CAD build for the part. Positions are in the model's coordinates, mm. Face numbers are marked on the shaded views. A direction names the side the tool comes from. Round coordinates to 2 decimals unless told otherwise and drop trailing zeros. Loops run counter-clockwise (first coordinate to the right, second up) from the corner with the lowest first, then second, coordinate; pieces in that order, holes last. Notation, with made-up numbers: (13, -16) - (31, -16) arc R4 cw to (31, -12) - close; hole circle Ø1 at (2.25, -20). An arc over 180 degrees is marked (long way). Use one line per item in the form item = value.
from build123d import *

# Parameters (mm, degrees)
F1_DEPTH       = 15
F3_DEPTH       = 112.001
F5_DEPTH       = 5
F7_DEPTH       = 112
F9_DEPTH       = 25
F12_DEPTH      = 15
F12_DEPTH_BACK = 5
F14_DEPTH      = 25
F15_R          = 3


# Not quite as in the source:
# - a pattern or mirror of a feature is missing from the dataset's text; its kind, count and spacing are read off the source's solid


with BuildPart() as f1:
    # F0 (on Top) → F1 (new body)
    with BuildSketch(Plane.XY):
        with BuildLine():
            Line((-56, 50), (-56, 0))
            Line((-56, 0), (56, 0))
            Line((56, 0), (56, 50))
            Line((56, 50), (36, 50))
            ThreePointArc((36, 50), (0, 14), (-36, 50))
            Line((-36, 50), (-56, 50))
        make_face()
    extrude(amount=F1_DEPTH)

    # F2 (on face) → F3 (cut, through all)
    with BuildSketch(Plane(origin=(-56, 0, 0), x_dir=(0, -1, 0), z_dir=(-1, 0, 0))):
        Polygon((-50, 12.5), (-50, 2.5), (-45, 7.5), align=None)
    extrude(amount=-F3_DEPTH, mode=Mode.SUBTRACT)

    # F4 (on face) → F5 (cut)
    with BuildSketch(Plane(origin=(0, 0, 0), x_dir=(1, 0, 0), z_dir=(0, 0, -1))):
        Polygon((-48.5, -45), (-48.5, -50), (-43.5, -50), (-43.5, -45), (-39.5, -41), (-52.5, -41), align=None)
        Polygon((43.5, -45), (43.5, -50), (48.5, -50), (48.5, -45), (52.5, -41), (39.5, -41), align=None)
    extrude(amount=-F5_DEPTH, mode=Mode.SUBTRACT)

    # F6 (on face) → F7 (join, through all)
    with BuildSketch(Plane(origin=(-56, 0, 0), x_dir=(0, -1, 0), z_dir=(-1, 0, 0))):
        Polygon((4.75, 7.5), (0, 12.25), (0, 2.75), align=None)
    extrude(amount=-F7_DEPTH)

    # F8 (on face) → F9 (cut)
    with BuildSketch(Plane(origin=(0, 0, 0), x_dir=(1, 0, 0), z_dir=(0, 0, -1))):
        Polygon((-47.5, 11.2829459831), (-47.5, 0), (-47.5, -5), (-42.5, -5), (-42.5, 0), (-42.5, 11.2829459831), align=None)
        Polygon((47.5, 11.2829459831), (42.5, 11.2829459831), (42.5, 0), (42.5, -5), (47.5, -5), (47.5, 0), align=None)
    extrude(amount=-F9_DEPTH, mode=Mode.SUBTRACT)

    # F11 (on mid) → F12 (cut, two sides)
    with BuildSketch(Plane(origin=(-45, 0, 0), x_dir=(0, -1, 0), z_dir=(-1, 0, 0))) as f12_sk:
        Polygon((0, 12.5), (-5, 7.5), (0, 2.5), (5, 7.5), align=None)
    f12 = extrude(amount=-F12_DEPTH, mode=Mode.SUBTRACT) + extrude(f12_sk.sketch, amount=F12_DEPTH_BACK, mode=Mode.SUBTRACT)

    # F12_copies: F12 across plane
    add(f12.mirror(Plane(origin=(0, 0, 0), x_dir=(0, 0, 1), z_dir=(1, 0, 0))), mode=Mode.SUBTRACT)

    # F13 (on face) → F14 (cut)
    with BuildSketch(Plane.XY.offset(15)):
        with BuildLine():
            Line((20, 15.0667409058), (20, 20.0667409058))
            ThreePointArc((20, 20.0667409058), (0, 14), (-20, 20.0667409058))
            Line((-20, 20.0667409058), (-20, 15.0667409058))
            ThreePointArc((-20, 15.0667409058), (0, 9), (20, 15.0667409058))
        make_face()
    extrude(amount=-F14_DEPTH, mode=Mode.SUBTRACT)

    # F15
    f15_edges = [f1.edges().sort_by_distance(p)[0] for p in [
        (-20, 20.066741, 7.5),
        (20, 20.066741, 7.5),
        (-20, 15.066741, 7.5),
        (20, 15.066741, 7.5),
    ]]
    fillet(f15_edges, radius=F15_R)


solid = f1.part
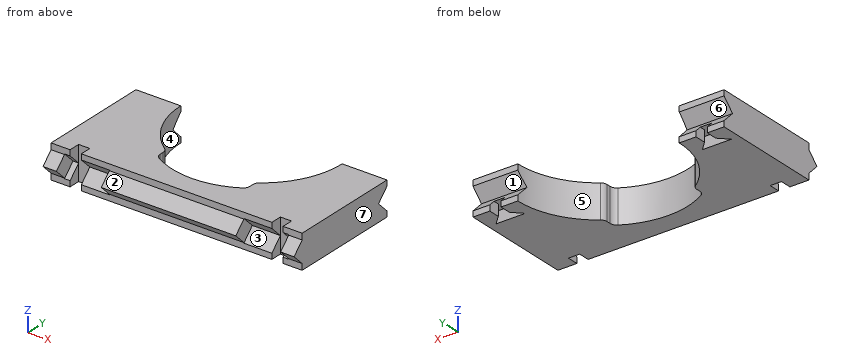
1) Tool access for the marked faces 1, 2, 3 and 4: list every direction of +Z, -Z, +X, -X, +Y, -Y with a clear straight run to the whole face (end or side of a thin tool).
Report:
face_1 = +X, -X, +Y
face_2 = +Z, +X, -X, -Y
face_3 = -Y
face_4 = +Z, -Z, +Y
2) Slice it at A-A (y = 2.5). Write the cut outline in (x, z), plus the area to 3 significant figures.
Report:
outline = (-56, 0) - (-47.5, 0) - (-47.5, 5) - (-50, 5) - (-50, 10) - (-47.5, 10) - (-47.5, 15) - (-56, 15) - close; (-42.5, 0) - (42.5, 0) - (42.5, 5) - (30, 5) - (30, 10) - (42.5, 10) - (42.5, 15) - (-42.5, 15) - (-42.5, 10) - (-30, 10) - (-30, 5) - (-42.5, 5) - close; (47.5, 0) - (56, 0) - (56, 15) - (47.5, 15) - (47.5, 10) - (50, 10) - (50, 5) - (47.5, 5) - close
area = 1,380 mm^2
3) Flat gauge pins, fed straight in: pin 1 (4 mm diameter, centred on x = -43, z = 3, fed in from +Y); pin 2 (1.5 mm diameter, centred on x = 45, z = 6, fed in from -Y); pin 3 (1 mm diameter, centred on x = 1.5, z = 13, fed in from +Y); pin 4 (8 mm diameter, centred on x = -10, y = 17, fed in from -Z). Where does each tip first touch, or does it go through?
Report:
pin_1 = 50
pin_2 = 5
pin_3 = 9.06
pin_4 = through
4) Two-plate mould, pull along X, no slides. Class the marked faces 5, 6 and 7: +X half, -X half, draft (parallel to the pull), parting line (faces both ways), or undercut.
Report:
face_5 = undercut
face_6 = draft
face_7 = +X half
5) Drill centre lines: probe 1 along X at (y, z) = (4.5, 1.25); probe 2 along Z at (x, y) = (32, 2); probe 3 along X at (y, z) = (39, 2.5). Where is each one in solid material? Low to high.
Report:
probe_1 = -56 to -47.5, -42.5 to 42.5, 47.5 to 56
probe_2 = 0 to 4.5, 10.5 to 15
probe_3 = -56 to -34.28, 34.28 to 56
6) Slice it at B-B (y = 38.5). Write the cut outline in (x, z).
Report:
outline = (-56, 0) - (-34.11, 0) - (-34.11, 15) - (-56, 15) - close; (34.11, 0) - (56, 0) - (56, 15) - (34.11, 15) - close
7) Slice it at C-C (x = 11). Write the cut outline in (y, z), plus the area to 3 significant figures.
Report:
outline = (-4.75, 7.5) - (0, 2.75) - (0, 0) - (10.72, 0) - (10.72, 15) - (0, 15) - (0, 12.25) - close
area = 183 mm^2
